Part print with two shaded views. Sizes in mm from the minimum x, y, z corner. A direction names the side the tool comes from. Round coordinates to 2 decimals unless told otherwise and drop trailing zeros. Order: outer loops, then holes, each group sorted by start corner. A loop starts at its lowest first (then second) coordinate and runs counter-clockwise, first axis right, second up. Notation, with made-up numbers: M 74,74.5 L 122,74.5 A9 ccw 122,87.5 Z; hole C -13.75,21 d10. An arc over 180 degrees is marked long. Put each result on its own line as item: value.
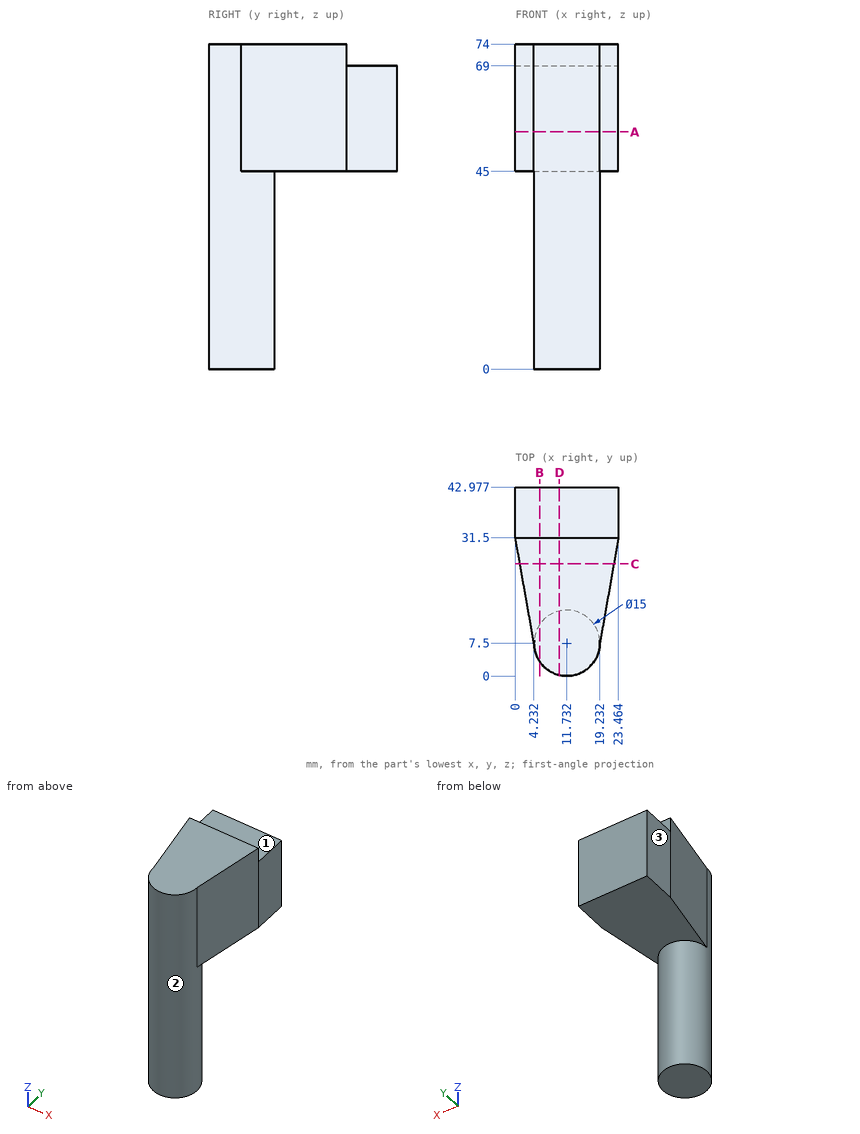
Item 1: Band-saw the part on B-B on x = 5.5. Give the cut face in (y, z).
Answers below:
outline: M 3.33,0 L 11.67,0 L 11.67,45 L 42.98,45 L 42.98,69 L 31.5,69 L 31.5,74 L 3.33,74 Z
Item 2: Band-saw the part on C-C on y = 25.5. Give the cut face in (x, z), and give its area (3 significant figures).
Answers below:
outline: M 1.06,45 L 22.41,45 L 22.41,74 L 1.06,74 Z
area: 619 mm²
Item 3: Probe line 1 along Z through (x, y) = (18.5, 21); line 2 along Z through (x, y) = (12, 38.5); line 3 along X through (y, z) = (4.5, 40.5) (1 decimal). List the from-to ranges inside material, lowest first. Write a range as [from, to].
Answers below:
line 1: [45, 74]
line 2: [45, 69]
line 3: [4.9, 18.6]
Item 4: Band-saw the part on A-A on z = 54. Give the cut face in (x, y), and give its area (3 significant figures).
Answers below:
outline: M 0,31.5 L 4.23,7.5 A7.5 ccw 19.23,7.5 L 23.46,31.5 L 23.46,42.98 L 0,42.98 Z
area: 819 mm²
Item 5: Band-saw the part on D-D on x = 10. Give the cut face in (y, z).
Answers below:
outline: M 0.2,0 L 14.8,0 L 14.8,45 L 42.98,45 L 42.98,69 L 31.5,69 L 31.5,74 L 0.2,74 Z
Item 6: Pin check, flat tips, straight feed: P1, Ø5, axis at x = 5.5, z = 59, coming from the -Y side (1 decimal); P2, Ø5.5, axis at x = 13.5, y = 39.5, coming from the +Z side; P3, Ø2, axis at x = 13.5, z = 28.5, coming from the +Y side. Stop position of each tip, or through.
Answers below:
P1: y = 1
P2: z = 69
P3: y = 14.96
Item 7: Tool access for the marked faces 1, 2 and 3: list every direction of +Z, -Z, +X, -X, +Y, -Y with a clear straight run to the whole face (end or side of a thin tool).
Answers below:
face 1: +Z, +X, -X, +Y
face 2: -Z
face 3: +Z, -Z, -X, +Y, -Y
